For this review, take the finished solid that the model builds, in its own axes (mm). A direction names the side the tool comes from. Give positions to 0.01 mm unless a question says otherwise; leave off trailing zeros. Loops run counter-clockwise (first coordinate to the right, second up) from the corner with the lowest first, then second, coordinate; pieces in that order, holes last.
```python
from build123d import *

# Parameters (mm, degrees)
SKETCH_W        = 143
SKETCH_H        = 142
PAD_DEPTH       = 2
SKETCH007_W     = 3
SKETCH007_H     = 4
PAD005_DEPTH    = 12
SKETCH008_W     = 103
SKETCH008_H     = 58
SKETCH008_W_2   = 101
SKETCH008_H_2   = 56
PAD006_DEPTH    = 2
SKETCH009_W     = 37
SKETCH009_H     = 38
PAD007_DEPTH    = 35
SKETCH010_W     = 37
SKETCH010_H     = 34.5
POCKET_DEPTH    = 3
SKETCH011_W     = 37
SKETCH011_H     = 22.5
POCKET001_DEPTH = 25
SKETCH013_W     = 27
SKETCH013_H     = 25
POCKET002_DEPTH = 45
SKETCH014_W     = 101
SKETCH014_H     = 56
POCKET003_DEPTH = 2.001
POCKET004_DEPTH = 2.001
FILLET_R        = 8
FILLET001_R     = 15


with BuildPart() as part:
    # Sketch → Pad (new body)
    with BuildSketch(Plane.XY):
        Rectangle(SKETCH_W, SKETCH_H)
    extrude(amount=PAD_DEPTH)

    # Sketch007 (on Face6 of Pad) → Pad005 (join)
    with BuildSketch(Plane.XY.offset(2)):
        with Locations((57.18826, -41.31823)):
            Rectangle(SKETCH007_W, SKETCH007_H)
        with Locations((51.63826, -41.31823)):
            Rectangle(SKETCH007_W, SKETCH007_H)
        with Locations((57.18826, -68.51823)):
            Rectangle(SKETCH007_W, SKETCH007_H)
        with Locations((51.63826, -68.51823)):
            Rectangle(SKETCH007_W, SKETCH007_H)
        Polygon((11.25, -65.67434), (14.25, -65.67434), (14.25, -70.67434), (11.25, -70.67434), (11.25, -69.17434), (12.75, -69.17434), (12.75, -67.17434), (11.25, -67.17434), align=None)
        Polygon((-14.25, -65.67434), (-11.25, -65.67434), (-11.25, -67.17434), (-12.75, -67.17434), (-12.75, -69.17434), (-11.25, -69.17434), (-11.25, -70.67434), (-14.25, -70.67434), align=None)
    extrude(amount=PAD005_DEPTH)

    # Sketch008 (on Face5 of Pad005) → Pad006 (join)
    with BuildSketch(Plane.XY.offset(2)):
        with Locations((0, 29)):
            Rectangle(SKETCH008_W, SKETCH008_H)
        with Locations((0, 29)):
            Rectangle(SKETCH008_W_2, SKETCH008_H_2, mode=Mode.SUBTRACT)
    extrude(amount=PAD006_DEPTH)

    # Sketch009 (on Face5 of Pad006) → Pad007 (join)
    with BuildSketch(Plane.XY.offset(2)):
        with Locations((0, -43.55182)):
            Rectangle(SKETCH009_W, SKETCH009_H)
    extrude(amount=PAD007_DEPTH)

    # Sketch010 (on Face48 of Pad007) → Pocket (cut)
    with BuildSketch(Plane.XY.offset(37)):
        with Locations((0, -43.55182)):
            Rectangle(SKETCH010_W, SKETCH010_H)
    extrude(amount=-POCKET_DEPTH, mode=Mode.SUBTRACT)

    # Sketch011 (on Face51 of Pocket) → Pocket001 (cut)
    with BuildSketch(Plane.XY.offset(34)):
        with Locations((0, -43.55182)):
            Rectangle(SKETCH011_W, SKETCH011_H)
    extrude(amount=-POCKET001_DEPTH, mode=Mode.SUBTRACT)

    # Sketch013 (on Face15 of Pocket001) → Pocket002 (cut)
    with BuildSketch(Plane.XZ.offset(62.55182)):
        with Locations((0, 19.5)):
            Rectangle(SKETCH013_W, SKETCH013_H)
    extrude(amount=-POCKET002_DEPTH, mode=Mode.SUBTRACT)

    # Sketch014 (on Face73 of Pocket002) → Pocket003 (cut, through all)
    with BuildSketch(Plane.XY.offset(2)):
        with Locations((0, 29)):
            Rectangle(SKETCH014_W, SKETCH014_H)
    extrude(amount=-POCKET003_DEPTH, mode=Mode.SUBTRACT)

    # Sketch015 (on Face5 of Pocket003) → Pocket004 (cut, through all)
    with BuildSketch(Plane.XY.offset(2)):
        with BuildLine():
            ThreePointArc((-24.986848, -19.655706), (-41.714005, -2.928549), (-58.441162, -19.655706))
            Line((-58.441162, -19.655706), (-58.441162, -47.734921))
            ThreePointArc((-58.441162, -47.734921), (-41.714005, -64.462078), (-24.986848, -47.734921))
            Line((-24.986848, -47.734921), (-24.986848, -19.655706))
        make_face()
        with BuildLine():
            ThreePointArc((-12.038252, -4.910588), (-20.155442, -13.027778), (-12.038252, -21.144968))
            Line((-12.038252, -21.144968), (56.984447, -21.144968))
            ThreePointArc((56.984447, -21.144968), (65.101637, -13.027778), (56.984447, -4.910588))
            Line((56.984447, -4.910588), (-12.038252, -4.910588))
        make_face()
        with BuildLine():
            ThreePointArc((-55.892961, 51.365669), (-61.221329, 56.694037), (-66.549697, 51.365669))
            Line((-66.549697, 51.365669), (-66.549697, 2.920796))
            ThreePointArc((-66.549697, 2.920796), (-61.221329, -2.407572), (-55.892961, 2.920796))
            Line((-55.892961, 2.920796), (-55.892961, 51.365669))
        make_face()
        with BuildLine():
            ThreePointArc((68.420184, 50.773804), (61.32185, 57.872138), (54.223516, 50.773804))
            Line((54.223516, 50.773804), (54.223516, 3.710121))
            ThreePointArc((54.223516, 3.710121), (61.32185, -3.388213), (68.420184, 3.710121))
            Line((68.420184, 3.710121), (68.420184, 50.773804))
        make_face()
    extrude(amount=-POCKET004_DEPTH, mode=Mode.SUBTRACT)

    # Fillet
    fillet_edges = [part.edges().sort_by_distance(p)[0] for p in [
        (16, -32.30182, 9),
        (-16, -32.30182, 9),
        (-16, -54.80182, 9),
        (16, -54.80182, 9),
    ]]
    fillet(fillet_edges, radius=FILLET_R)

    # Fillet001
    fillet001_edges = [part.edges().sort_by_distance(p)[0] for p in [
        (-71.5, -71, 1),
        (71.5, -71, 1),
        (71.5, 71, 1),
        (-71.5, 71, 1),
    ]]
    fillet(fillet001_edges, radius=FILLET001_R)


solid = part.part
```
Q1. Consider section B-B on y = -28.5. Give the boundary of the cut face in (x, z).
Answers:
outline: (-71.5, 0) - (-58.44, 0) - (-58.44, 2) - (-71.5, 2) - close; (-24.99, 0) - (71.5, 0) - (71.5, 2) - (18.5, 2) - (18.5, 34) - (-18.5, 34) - (-18.5, 2) - (-24.99, 2) - close; hole (-13.5, 7) - (13.5, 7) - (13.5, 32) - (-13.5, 32) - close
Q2. Machinability: for faces 1 (the flat face through (53.138, -41, 8)), 2 (the flat face through (0, -59, 32)), 3 (the flat face through (-16, -44, 9)), 4 (the flat face through (58.688, -69, 8)), which of the approach directions +Z, -Z, +X, -X, +Y, -Y give a long, thin tool a straight path to every point of the face, cutting with its end or side? Answer none if there is none.
Answers:
face 1: +Z, +Y, -Y
face 2: +Y, -Y
face 3: +Z, -X
face 4: +Z, +X, +Y, -Y
Q3. Consider section D-D on x = 33. Give the boundary of the cut face in (y, z), plus the area to 3 significant figures.
Answers:
outline: (-71, 0) - (-21.14, 0) - (-21.14, 2) - (-71, 2) - close; (-4.91, 0) - (1, 0) - (1, 4) - (0, 4) - (0, 2) - (-4.91, 2) - close; (57, 0) - (71, 0) - (71, 2) - (58, 2) - (58, 4) - (57, 4) - close
area: 144 mm2
Q4. For pin 1 Ø8 at (y, z) = (20, 7) entering from +X; pin 2 Ø3 at (y, z) = (-68, 5) entering from -X; pin 3 Ø12 at (x, y) = (-23, -46.5) entering from +Z, all flat-tipped, find the tip position at first contact; note any pin that passes through.
Answers:
pin 1: stops at x = 51.5
pin 2: stops at x = -14.25
pin 3: stops at z = 9.89
Q5. Consider section A-A on z = 24. Give the boundary of the cut face in (x, y).
Answers:
outline: (-18.5, -62.55) - (-13.5, -62.55) - (-13.5, -54.8) - (-18.5, -54.8) - close; (-18.5, -32.3) - (-13.5, -32.3) - (-13.5, -24.55) - (-18.5, -24.55) - close; (13.5, -62.55) - (18.5, -62.55) - (18.5, -54.8) - (13.5, -54.8) - close; (13.5, -32.3) - (18.5, -32.3) - (18.5, -24.55) - (13.5, -24.55) - close
Q6. For probe 1 along Y at (x, z) = (-6, 3.5); probe 2 along Y at (x, z) = (15, 31.5); probe 3 along Z at (x, y) = (53, 2), list the stretches that pass through material, from the lowest coordinate up.
Answers:
probe 1: y = -62.55 to -24.55, 0 to 1, 57 to 58
probe 2: y = -62.55 to -54.8, -32.3 to -24.55
probe 3: z = 0 to 2
Q7. Mouldability with a two-part tool opening along X and no side actions: class faces 5 (the cylindrical face through (66.99, 66.72, 1.01)), 6 (the cylindrical face through (16.035, -52.521, 11.406)), 7 (the cylindrical face through (-67.22, 66.49, 1.01)), 8 (the flat face through (-1, 1, 2)) as +X half, -X half, draft (parallel to the pull), parting line (faces both ways), or undercut.
Answers:
face 5: +X half
face 6: draft
face 7: -X half
face 8: undercut
Q8. Consider section C-C on y = 35. Give the boundary of the cut face in (x, z), plus the area to 3 significant figures.
Answers:
outline: (-71.5, 0) - (-66.55, 0) - (-66.55, 2) - (-71.5, 2) - close; (-55.89, 0) - (-50.5, 0) - (-50.5, 4) - (-51.5, 4) - (-51.5, 2) - (-55.89, 2) - close; (50.5, 0) - (54.22, 0) - (54.22, 2) - (51.5, 2) - (51.5, 4) - (50.5, 4) - close; (68.42, 0) - (71.5, 0) - (71.5, 2) - (68.42, 2) - close
area: 38.3 mm2
